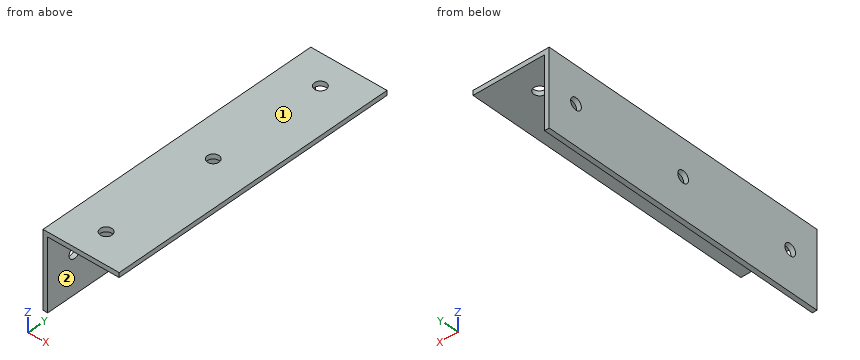
from build123d import *

# Parameters (mm, degrees)
EXTRUDE_1_DEPTH     = 250
SKETCH_6_R          = 5
CUT_EXTRUDE_1_DEPTH = 10
SKETCH_7_R          = 5
CUT_EXTRUDE_2_DEPTH = 10


with BuildPart() as part:
    # Эскиз1 → Вытянуть-Тонкостенный1 (new body)
    with BuildSketch(Plane(origin=(0, 0, 0), x_dir=(1, 0, 0), z_dir=(0, 1, 0))):
        Polygon((0, 65), (0, 0), (65, 0), (65, 4), (4, 4), (4, 65), align=None)
    extrude(amount=EXTRUDE_1_DEPTH)

    # Эскиз6 → Вырез-Вытянуть1 (cut)
    with BuildSketch(Plane.ZY):
        with Locations((-31, 25)):
            Circle(SKETCH_6_R)
        with Locations((-31, 125)):
            Circle(SKETCH_6_R)
        with Locations((-31, 225)):
            Circle(SKETCH_6_R)
    extrude(amount=-CUT_EXTRUDE_1_DEPTH, mode=Mode.SUBTRACT)

    # Эскиз7 → Вырез-Вытянуть2 (cut)
    with BuildSketch(Plane.XY):
        with Locations((31, 25)):
            Circle(SKETCH_7_R)
        with Locations((31, 125)):
            Circle(SKETCH_7_R)
        with Locations((31, 225)):
            Circle(SKETCH_7_R)
    extrude(amount=-CUT_EXTRUDE_2_DEPTH, mode=Mode.SUBTRACT)


solid = part.part
Verification items for the finished model (mm, model axes). Face numbers are marked on the shaded views. A direction names the side the tool comes from. Coordinates: 2 decimals unless noted, no trailing zeros. Loops run counter-clockwise (first coordinate to the right, second up) from the corner with the lowest first, then second, coordinate; pieces in that order, holes last. Notation, with made-up numbers: (52, -5) -> (79, -5) arc R20 ccw to (79, 5) -> close; hole circle Ø4 at (-17.75, -3.75). An arc over 180 degrees is marked (long way). Answer as a JSON object with one key per item and string values. Group by question number.
Item 1: Sectioned sample at B-B on y = 25. Record the boundary of the cut face in (x, z), plus the area to 3 significant figures.
Item 2: Scan lines: probe 1 along Y at (x, z) = (2, -31); probe 2 along Z at (x, y) = (7.5, 167); probe 3 along X at (y, z) = (83.5, -58). Record each from-to range of solid material in increasing order.
Item 3: Sectioned sample at A-A on x = 31. Record the boundary of the cut face in (y, z).
Item 4: Sectioned sample at D-D on x = 10. Record the boundary of the cut face in (y, z).
Item 5: Sectioned sample at C-C on z = -29.5. Record the boundary of the cut face in (x, y).
Item 6: Tool access check on the marked faces 1 and 2. Record the directions out of +Z, -Z, +X, -X, +Y, -Y that give a thin tool (end or side, any length) a straight path to the whole face; none if there is none.
Item 7: Depth check by flat-ended pin: pin 1 (9 mm diameter, centred on x = 31, y = 225, fed in from +Z); pin 2 (1.5 mm diameter, centred on y = 89, z = -28.5, fed in from +X); pin 3 (3 mm diameter, centred on x = 37, y = 172, fed in from -Z); pin 4 (11.5 mm diameter, centred on y = 25, z = -31, fed in from -X). Enter the tip coordinate at first touch or a pass-through.
Evaluation:
{
 "1": {"outline": "(0, -65) -> (4, -65) -> (4, -36) -> (0, -36) -> close; (0, -26) -> (4, -26) -> (4, -4) -> (26, -4) -> (26, 0) -> (0, 0) -> close; (36, -4) -> (65, -4) -> (65, 0) -> (36, 0) -> close", "area": "424 mm²"},
 "2": {"probe 1": "y = 0 to 20, 30 to 120, 130 to 220, 230 to 250", "probe 2": "z = -4 to 0", "probe 3": "x = 0 to 4"},
 "3": {"outline": "(0, -4) -> (20, -4) -> (20, 0) -> (0, 0) -> close; (30, -4) -> (120, -4) -> (120, 0) -> (30, 0) -> close; (130, -4) -> (220, -4) -> (220, 0) -> (130, 0) -> close; (230, -4) -> (250, -4) -> (250, 0) -> (230, 0) -> close"},
 "4": {"outline": "(0, -4) -> (250, -4) -> (250, 0) -> (0, 0) -> close"},
 "5": {"outline": "(0, 0) -> (4, 0) -> (4, 20.23) -> (0, 20.23) -> close; (0, 29.77) -> (4, 29.77) -> (4, 120.23) -> (0, 120.23) -> close; (0, 129.77) -> (4, 129.77) -> (4, 220.23) -> (0, 220.23) -> close; (0, 229.77) -> (4, 229.77) -> (4, 250) -> (0, 250) -> close"},
 "6": {"face 1": "+Z, +X, -X, +Y, -Y", "face 2": "-Z, +X, +Y, -Y"},
 "7": {"pin 1": "passes through", "pin 2": "stops at x = 4", "pin 3": "stops at z = -4", "pin 4": "stops at x = 0"}
}
